Print and shaded views of the part. All mm, measured from the part's lowest x, y and z. A direction names the side the tool comes from. Round coordinates to 2 decimals unless told otherwise and drop trailing zeros. Order: outer loops, then holes, each group sorted by start corner. A loop starts at its lowest first (then second) coordinate and runs counter-clockwise, first axis right, second up. Notation, with made-up numbers: (56.5, 0.5) - (78.5, 0.5) arc R17 cw to (78.5, 13.5) - close; hole circle Ø1 at (-33.5, 73.5). An arc over 180 degrees is marked (long way). Write item = value, one per line.
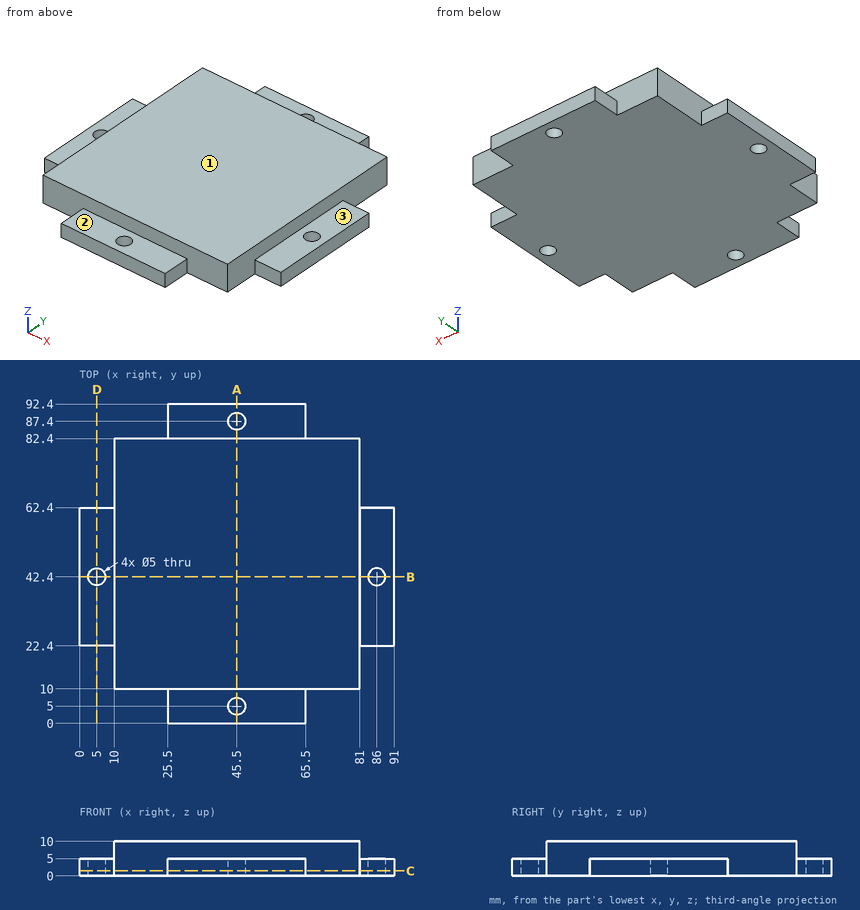
(1) Probe line 1 along Y through (x, z) = (45.5, 2.7); line 2 along X through (y, z) = (21, 7.5); line 3 along Y through (x, z) = (77.5, 8). List the from-to ranges inside material, lowest first.
Solved:
line_1 = 0 to 2.5, 7.5 to 84.9, 89.9 to 92.4
line_2 = 10 to 81
line_3 = 10 to 82.4
(2) Band-saw the part on A-A on x = 45.5. List the corners of the cut face in (y, z).
Solved:
outline = (0, 0) - (2.5, 0) - (2.5, 5) - (0, 5) - close; (7.5, 0) - (84.9, 0) - (84.9, 5) - (82.4, 5) - (82.4, 10) - (10, 10) - (10, 5) - (7.5, 5) - close; (89.9, 0) - (92.4, 0) - (92.4, 5) - (89.9, 5) - close
(3) Band-saw the part on C-C on z = 1.5. List the corners of the cut face in (x, y).
Solved:
outline = (0, 22.4) - (10, 22.4) - (10, 10) - (25.5, 10) - (25.5, 0) - (65.5, 0) - (65.5, 10) - (81, 10) - (81, 22.4) - (91, 22.4) - (91, 62.4) - (81, 62.4) - (81, 82.4) - (65.5, 82.4) - (65.5, 92.4) - (25.5, 92.4) - (25.5, 82.4) - (10, 82.4) - (10, 62.4) - (0, 62.4) - close; hole circle Ø5 at (5, 42.4); hole circle Ø5 at (45.5, 5); hole circle Ø5 at (45.5, 87.4); hole circle Ø5 at (86, 42.4)
(4) Drop flat-ended pins along their axis: pin 1 (4.5 mm diameter, centred on x = 45.5, y = 87.4, fed in from +Z); pin 2 (5 mm diameter, centred on x = 48.5, y = 7, fed in from +Z); pin 3 (4 mm diameter, centred on y = 7, z = 2, fed in from +X); pin 4 (1 mm diameter, centred on x = 35.5, z = 7, fed in from -Y). Give the stop position or say it passes through.
Solved:
pin_1 = through
pin_2 = 5
pin_3 = 65.5
pin_4 = 10
(5) Band-saw the part on B-B on y = 42.4. List the corners of the cut face in (x, z), plus the area to 3 significant figures.
Solved:
outline = (0, 0) - (2.5, 0) - (2.5, 5) - (0, 5) - close; (7.5, 0) - (83.5, 0) - (83.5, 5) - (81, 5) - (81, 10) - (10, 10) - (10, 5) - (7.5, 5) - close; (88.5, 0) - (91, 0) - (91, 5) - (88.5, 5) - close
area = 760 mm²
(6) Tool access for the marked faces 1, 2 and 3: list every direction of +Z, -Z, +X, -X, +Y, -Y with a clear straight run to the whole face (end or side of a thin tool).
Solved:
face_1 = +Z, +X, -X, +Y, -Y
face_2 = +Z, +X, -X, -Y
face_3 = +Z, +X, +Y, -Y
(7) Band-saw the part on D-D on x = 5. List the corners of the cut face in (y, z).
Solved:
outline = (22.4, 0) - (39.9, 0) - (39.9, 5) - (22.4, 5) - close; (44.9, 0) - (62.4, 0) - (62.4, 5) - (44.9, 5) - close
